Geometry: see drawing. Coordinates: mm, zero at the bounding-box minimum. Give positions to 0.01 mm unless a question says otherwise; leave off trailing zeros. Loops run counter-clockwise (first coordinate to the right, second up) from the corner with the lowest first, then second, coordinate; pieces in that order, holes last. Notation, with made-up numbers: (-8, 85) -> (26, 85) arc R28 ccw to (26, 123) -> close; hole circle Ø7 at (34, 71.5). An arc over 180 degrees is marked (long way). Return JSON: item names as keys, results as strings. Group by question number.
(1) Ray query, line 1 (Y direction, x = 10.5, z = 5.5); line 2 (Y direction, x = 10, z = 5.5) (1 decimal); line 3 (X direction, y = 106.5, z = 10.5). Return the intervals inside material, ascending. Write a range as from..to.
(2) Cut plane B-B on y = 13. Return loops of the section in (x, z).
(3) Cut plane A-A on x = 10. Return loops of the section in (y, z) (1 decimal), then the cut area to 3 significant figures.
(4) Draft query along X for the marked faces 1, 2 and 3. Return one class per face: released by +X, released by -X, zero draft, split by the parting line, or undercut.
(5) Cut plane C-C on z = 2.25. Return loops of the section in (x, y) (1 decimal).
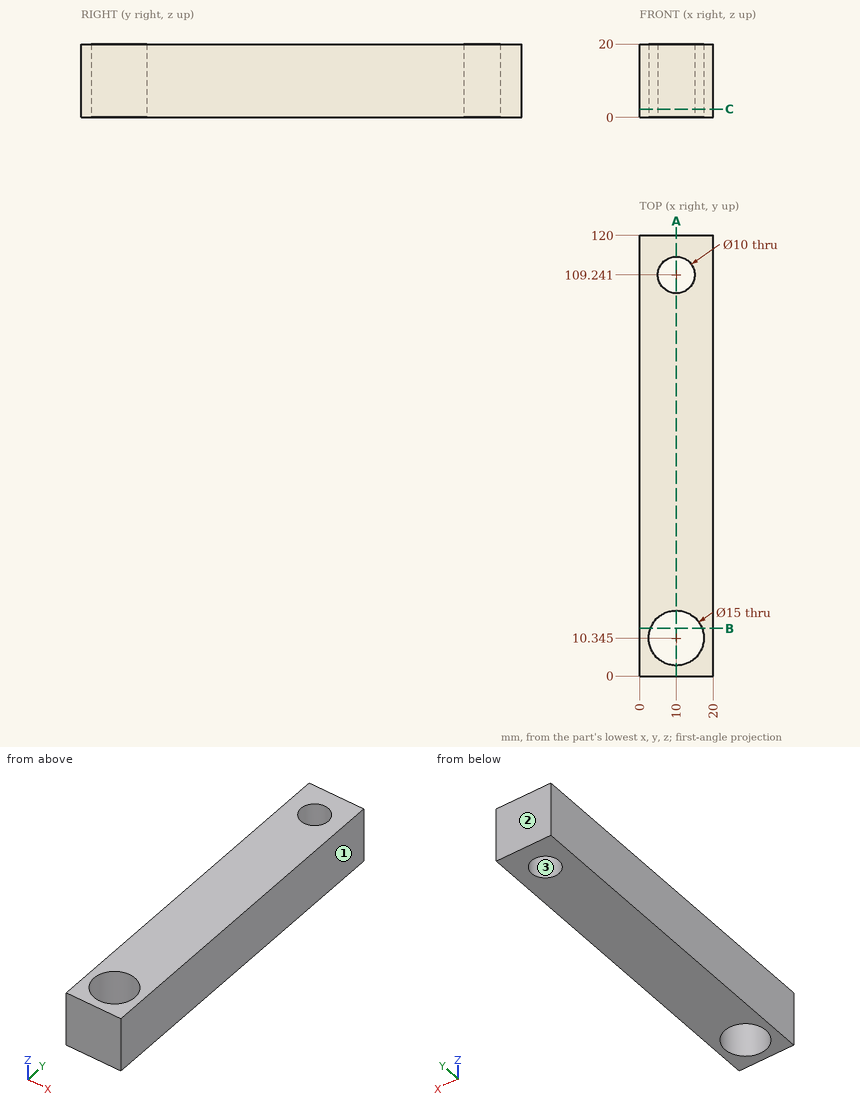
Answers:
{
 "1": {"line 1": "0..2.86, 17.83..104.27, 114.22..120", "line 2": "0..2.8, 17.8..104.2, 114.2..120", "line 3": "0..5.82, 14.18..20"},
 "2": {"outline": "(0, 0) -> (2.99, 0) -> (2.99, 20) -> (0, 20) -> close; (17.01, 0) -> (20, 0) -> (20, 20) -> (17.01, 20) -> close"},
 "3": {"outline": "(0, 0) -> (2.8, 0) -> (2.8, 20) -> (0, 20) -> close; (17.8, 0) -> (104.2, 0) -> (104.2, 20) -> (17.8, 20) -> close; (114.2, 0) -> (120, 0) -> (120, 20) -> (114.2, 20) -> close", "area": "1,900 mm²"},
 "4": {"face 1": "released by +X", "face 2": "zero draft", "face 3": "undercut"},
 "5": {"outline": "(0, 0) -> (20, 0) -> (20, 120) -> (0, 120) -> close; hole circle Ø15 at (10, 10.3); hole circle Ø10 at (10, 109.2)"}
}
